Design review of the part built by this model. Coordinates are the model's own, in mm. A direction names the side the tool comes from. Give positions to 0.01 mm unless a question says otherwise; leave off trailing zeros. Loops run counter-clockwise (first coordinate to the right, second up) from the corner with the lowest first, then second, coordinate; pieces in that order, holes last. Notation, with made-up numbers: (-3, -33) -> (11, -33) arc R26 cw to (11, -2) -> close; hole circle Ø4 at (22.25, -4.5). An arc over 180 degrees is marked (long way). Use a Markdown table: item, result. Add a question column.
1. For pin 1 Ø1 at (x, y) = (111.5, 201.5) entering from -Z; pin 2 Ø5 at (x, z) = (111.56, -6.5) entering from -Y; pin 3 Ø7 at (x, z) = (111.56, -31.5) entering from +Y; pin 4 Ø5 at (x, y) = (115.5, 203) entering from -Z, all flat-tipped, find the tip position at first contact; note any pin that passes through.
2. Add section B-B (x = 113.25). State the section outline as (y, z) points.
3. To check wall thickness, follow line 1 (X direction, y = 197.7, z = -6.5); line 2 (Y direction, x = 109.25, z = -36); line 3 (Z direction, x = 117.75, y = 209). State the ranges of each line that lie inside material, in increasing order.
4. Add section C-C (y = 202.5). State the section outline as (x, z) points, and give its area (3 significant figures).
5. Draft analysis for pull direction Y (two halves, no side actions). For faces 4 (the flat face through (111, 195.484, -19)), 5 (the flat face through (101.606, 201, -15)), 6 (the flat face through (106.99, 202.41, -3.64)), 7 (the cylindrical face through (111.42, 212.82, -19.83)), state which applies: pulls with the +Y half, pulls with the -Y half, needs draft (parallel to the pull), parting line crosses it, or undercut.
6. Add section A-A (z = -31.5). State the section outline as (x, y) points.
7. For faces 1 (the cylindrical face through (111.5, 202.9, -26.7)), 2 (the cylindrical face through (108.628, 196.963, -5.85)), 3 (the flat face through (114, 198.484, -9)), list the 3-axis set-ups (+Z, -Z, +X, -X, +Y, -Y) from which the entire face can be reached by the end or side of a thin tool; tool diameter is ignored.
8. Add section D-D (x = 104.25). State the section outline as (y, z) points, and give its area (3 significant figures).
```python
from build123d import *

# Parameters (mm, degrees)
BOSS_EXTRUDE1_DEPTH = 38
SKETCH2_R           = 6.39
BOSS_EXTRUDE2_DEPTH = 19.9


with BuildPart() as part:
    # Sketch1 → Boss-Extrude1 (new body)
    with BuildSketch(Plane.XY):
        Polygon((101.60617691, 195.484265545), (108.51617691, 195.484265545), (114.604851948, 195.484265545), (121.50617691, 195.484265545), (121.50617691, 198.484265545), (101.60617691, 198.484265545), align=None)
    extrude(amount=-BOSS_EXTRUDE1_DEPTH)

    # Sketch2 → Boss-Extrude2 (add)
    with BuildSketch(Plane.ZY.offset(-101.60617691)):
        with BuildLine():
            Line((-28.843974353, 198.484265545), (-27.399359103, 207.788399993))
            ThreePointArc((-27.399359103, 207.788399993), (-21.484497631, 214.613058291), (-12.764937605, 212.261288734))
            Line((-12.764937605, 212.261288734), (0, 198.484265545))
            Line((0, 198.484265545), (-28.843974353, 198.484265545))
        make_face()
        with Locations((-19, 206.484265545)):
            Circle(SKETCH2_R, mode=Mode.SUBTRACT)
    extrude(amount=-BOSS_EXTRUDE2_DEPTH)

    # Sketch3 → Cut-Revolve1 (revolve, cut)
    with BuildSketch(Plane.ZY.offset(-111.55617691)):
        Polygon((-26.7, 211.670017018), (-26.7, 198.484265545), (-28.5, 198.484265545), (-28.5, 189.906068288), (-31.5, 189.906068288), (-31.5, 211.670017018), align=None)
    cut_revolve1 = revolve(axis=Axis((111.55617691, 189.906068288, -31.5), (0, 1, 0)), mode=Mode.SUBTRACT)

    # Mirror1: Cut-Revolve1 across plane
    add(cut_revolve1.mirror(Plane(origin=(0, 0, -19), x_dir=(1, 0, 0), z_dir=(0, 0, -1))), mode=Mode.SUBTRACT)


solid = part.part
```
Taken from the geometry:
| question | item | result |
|---|---|---|
| 1 | pin 1 | stops at z = -26.73 |
| 1 | pin 2 | passes through |
| 1 | pin 3 | stops at y = 198.48 |
| 1 | pin 4 | stops at z = -28.53 |
| 2 | outline | (195.48, -38) -> (198.48, -38) -> (198.48, -33.98) -> (195.48, -33.98) -> close; (195.48, -29.02) -> (198.48, -29.02) -> (198.48, -27.01) -> (209.33, -27.01) arc R8.5 ccw to (212.26, -12.76) -> (210.35, -10.99) -> (198.48, -10.99) -> (198.48, -8.98) -> (195.48, -8.98) -> close; (195.48, -4.02) -> (198.48, -4.02) -> (198.48, -2.01) -> (200.65, -2.01) -> (198.48, 0) -> (195.48, 0) -> close; hole circle Ø12.78 at (206.48, -19) |
| 3 | line 1 | x = 101.61 to 108.56, 114.56 to 121.51 |
| 3 | line 2 | y = 195.48 to 198.48 |
| 3 | line 3 | z = -27.12 to -24.87, -13.13 to -9.74 |
| 4 | outline | (101.61, -28.22) -> (108.05, -28.22) arc R4.8 cw to (115.06, -28.22) -> (121.51, -28.22) -> (121.51, -24) -> (101.61, -24) -> close; (101.61, -14) -> (121.51, -14) -> (121.51, -3.72) -> (115.47, -3.72) arc R4.8 cw (long way) to (107.64, -3.72) -> (101.61, -3.72) -> close |
| 4 | area | 220 mm^2 |
| 5 | face 4 | pulls with the -Y half |
| 5 | face 5 | needs draft |
| 5 | face 6 | pulls with the +Y half |
| 5 | face 7 | undercut |
| 6 | outline | (101.61, 195.48) -> (108.56, 195.48) -> (108.56, 198.48) -> (101.61, 198.48) -> close; (114.56, 195.48) -> (121.51, 195.48) -> (121.51, 198.48) -> (114.56, 198.48) -> close |
| 7 | face 1 | -Z, +Y |
| 7 | face 2 | +Y, -Y |
| 7 | face 3 | +Y |
| 8 | outline | (195.48, -38) -> (198.48, -38) -> (198.48, -28.84) -> (207.79, -27.4) arc R8.5 ccw to (212.26, -12.76) -> (198.48, 0) -> (195.48, 0) -> close; hole circle Ø12.78 at (206.48, -19) |
| 8 | area | 302 mm^2 |
